CAD build for the part. Positions are in the model's coordinates, mm. Face numbers are marked on the shaded views. A direction names the side the tool comes from. Coordinates: 2 decimals unless noted, no trailing zeros. Loops run counter-clockwise (first coordinate to the right, second up) from the corner with the lowest first, then second, coordinate; pieces in that order, holes last. Notation, with made-up numbers: M 67,77.5 L 111,77.5 A30 cw 111,111.5 Z; hole C 33.25,54 d1. An arc over 180 degrees is marked long. Answer as a JSON object with one key per item and string values. Group by question number.
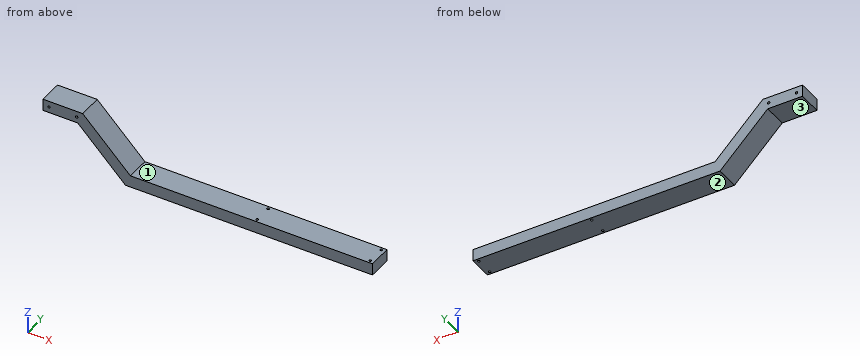
Autodesk Inventor part; units mm, degrees
ref_plane "YZ Plane" through (0, 0, 0) normal (1, 0, 0) x (0, 1, 0)
ref_plane "XZ Plane" through (0, 0, 0) normal (0, 1, 0) x (-1, 0, 0)
ref_plane "XY Plane" through (0, 0, 0) normal (0, 0, 1) x (1, 0, 0)
sketch "草圖1" plane through (0, 0, 0) normal (0, 0, 1) x (1, 0, 0)
  line L0 (-10, -30) -> (10, 30) construction
  line L1 (10, -30) -> (-10, 30) construction
  line L2 (10, 30) -> (-600, 30)
  line L3 (-600, 30) -> (-600, -30)
  line L4 (-600, -30) -> (10, -30)
  line L5 (10, -30) -> (10, 30)
  circle A0 centre (0, 22.5) radius 3
  circle A1 centre (0, -22.5) radius 3
  circle A2 centre (-285, 22.5) radius 3
  circle A3 centre (-285, -22.5) radius 3
  point P0 (0, 0)
  dimension "d0" = 20
  dimension "d1" = 60
  dimension "d2" = 610
  dimension "d4" = 6
  dimension "d5" = 6
  dimension "d8" = 6
  dimension "d9" = 6
extrude "擠出1" add sketch "草圖1" along normal blind 30
sketch "草圖2" plane through (-600, -30, 0) normal (0, -1, 0) x (1, 0, 0)
  line L0 (0, 30) -> (-120.2082, 150.2082)
  line L1 (0, 30) -> (170, 30) construction
  line L2 (-120.2082, 150.2082) -> (-141.4214, 128.9949)
  line L3 (-141.4214, 128.9949) -> (-12.4264, 0)
  line L4 (0, 0) -> (610, 0)
  line L5 (-12.4264, 0) -> (0, 0)
  line L6 (0, 0) -> (0, 30)
  line L7 (-120.2082, 150.2082) -> (-220.2082, 150.2082)
  line L8 (-220.2082, 150.2082) -> (-220.2082, 120.2082)
  line L9 (-220.2082, 120.2082) -> (-132.6346, 120.2082)
  point P0 (600, 0)
  dimension "d13" = 170
  dimension "d14" = 135
  dimension "d15" = 30
  dimension "d16" = 100
  dimension "d17" = 30
extrude "擠出2" add sketch "草圖2" against normal blind 60
sketch "草圖3" plane through (10, 30, 30) normal (0, 1, 0) x (1, 0, 0)
  line L0 (-830.2082, -90.2082) -> (-830.2082, -120.2082)
  circle A0 centre (-815.2082, -105.2082) radius 3
  circle A1 centre (-745.2082, -105.2082) radius 3
  point P0 (-10, 30)
  dimension "d22" = 6
  dimension "d23" = 6
extrude "擠出3" cut sketch "草圖3" along normal through all both and the other way through all
properties part number "DOF2"
Item 1: Pin check, flat tips, straight feed: pin 1 (6 mm diameter, centred on x = -644, y = 16, fed in from -Z); pin 2 (2 mm diameter, centred on x = -563, y = -3.5, fed in from -Z); pin 3 (18 mm diameter, centred on x = -312, y = 3.5, fed in from +Z); pin 4 (6 mm diameter, centred on y = -14, z = 38, fed in from +X). Stop position of each tip, or through.
Item 2: Slice it at A-A, the plane y = -8.5. Write the cut outline in (x, z).
Item 3: Slice it at B-B, the plane x = -125.5. Write the cut outline in (y, z).
Item 4: Tool access for the marked faces 1, 2 and 3: list every direction of +Z, -Z, +X, -X, +Y, -Y with a clear straight run to the whole face (end or side of a thin tool).
Item 5: Drill centre lines: L1, parallel to Y at x = -285, z = 21; L2, parallel to X at y = -22, z = 10; L3, parallel to Z at x = -184.5, y = -12.5. Where is each one in solid material? Low to high. Write a range as from..to.
Item 6: Slice it at C-C, the plane z = 48.5. Write the cut outline in (x, y), then the cut area to 3 significant figures.
Computed:
{
 "1": {"pin 1": "z = 28.57", "pin 2": "z = 0", "pin 3": "z = 30", "pin 4": "x = -605"},
 "2": {"outline": "M -820.21,120.21 L -732.63,120.21 L -612.43,0 L 10,0 L 10,30 L -600,30 L -720.21,150.21 L -820.21,150.21 Z; hole C -805.21,135.21 d6; hole C -735.21,135.21 d6"},
 "3": {"outline": "M -30,0 L 30,0 L 30,30 L -30,30 Z"},
 "4": {"face 1": "+Z, +X, +Y, -Y", "face 2": "-Z, +X, -X, +Y, -Y", "face 3": "-Z, -X, +Y, -Y"},
 "5": {"L1": "-30..-25.5, -19.5..19.5, 25.5..30", "L2": "-622.43..-287.96, -282.04..-2.96, 2.96..10", "L3": "0..30"},
 "6": {"outline": "M -660.93,-30 L -618.5,-30 L -618.5,30 L -660.93,30 Z", "area": "2,550 mm2"}
}
